```python
from build123d import *

# Parameters (mm, degrees)
BOSS_EXTRUDE3_DEPTH = 117
SKETCH3_W           = 2.281994321
SKETCH3_H           = 23.79794077
SKETCH3_W_2         = 80.521799592
SKETCH3_H_2         = 88.019780931
CUT_EXTRUDE1_DEPTH  = 117
SKETCH4_W           = 94.510648664
SKETCH4_H           = 87.992672894
CUT_EXTRUDE2_DEPTH  = 117


with BuildPart() as part:
    # Sketch2 → Boss-Extrude3 (new body)
    with BuildSketch(Plane(origin=(0, 0, 0), x_dir=(1, 0, 0), z_dir=(0, 1, 0))):
        Polygon((-826.128986822, -44.396477746), (-786.035151567, -12.233698412), (-620.035151567, -12.233698412), (-580.129096878, -44.629173391), (-580.129096878, -114.629173391), (-664.384727068, -191.421027004), (-742.086028689, -191.421027004), (-826.128986822, -114.396477746), align=None)
    extrude(amount=BOSS_EXTRUDE3_DEPTH)

    # Sketch3 → Cut-Extrude1 (cut)
    with BuildSketch(Plane(origin=(-206.167073408, 0, -226.205461612), x_dir=(0.7390844753537593, 0, -0.6736127509860976), z_dir=(0.6736127509860976, 0, 0.7390844753537593))):
        with Locations((-598.858942552, 121.091844218)):
            Rectangle(SKETCH3_W, SKETCH3_H)
        with Locations((-562.673032613, 60.618994727)):
            Rectangle(SKETCH3_W_2, SKETCH3_H_2)
    extrude(amount=-CUT_EXTRUDE1_DEPTH, mode=Mode.SUBTRACT)

    # Sketch4 → Cut-Extrude2 (cut)
    with BuildSketch(Plane(origin=(-434.116139586, 0, 473.672418674), x_dir=(0.7372189309889005, 0, 0.6756539408540315), z_dir=(-0.6756539408540315, 0, 0.7372189309889005))):
        with Locations((-474.328289605, 59.966544548)):
            Rectangle(SKETCH4_W, SKETCH4_H)
    extrude(amount=-CUT_EXTRUDE2_DEPTH, mode=Mode.SUBTRACT)


solid = part.part
```
Can you work these out from the model? Positions are in its coordinate system, mm. A direction names the side the tool comes from. Give positions to 0.01 mm unless a question says otherwise; leave off trailing zeros. Loops run counter-clockwise (first coordinate to the right, second up) from the corner with the lowest first, then second, coordinate; pieces in that order, holes last. Notation, with made-up numbers: M 84,23.5 L 133,23.5 A26 ccw 133,50.5 Z; hole C -3,54.5 d9. An arc over 180 degrees is marked long. Use one line per item in the form item = value. Start each with the question number.
(1) I want a section at D-D, the plane z = 140.5. Write out the boundary of the cut face in (x, y).
(2) Thinking about a two-plate mould opening in Z: for faces 1 (the flat face through (-754, 103.963, 120)), 2 (the flat face through (-703, 58, 191.421)), 3 (the flat face through (-688.03, 61.24, 54.67)), 4 (the flat face through (-826.129, 58, 80)), which applies, released by +Z, released by -Z, zero draft, split by the parting line, or undercut?
(3) I'm going to push flat-ended pins straight in: P1, Ø10, axis at x = -625, z = 56.5, coming from the -Y side; P2, Ø6, axis at y = 27, z = 39.5, coming from the +X side; P3, Ø12, axis at x = -637.5, y = 42, coming from the +Z side. Where does each tip first touch, or does it pass through?
(4) I want a section at A-A, the plane z = 76.5. Write out the boundary of the cut face in (x, y).
(5) I want a section at B-B, the plane x = -716. Write out the boundary of the cut face in (y, z).
(6) I want a section at C-C, the plane y = 40. Write out the boundary of the cut face in (x, z), and give its area (3 significant figures).
(7) On a 3-axis mill with a long thin cutter (end or side, diameter ignored), from which of +Z, -Z, +X, -X, +Y, -Y can I reach the whole of each face in a straight line? I mean faces 5 (the flat face through (-701, 0, 101)), 6 (the flat face through (-661, 104.629, 111)), 7 (the flat face through (-688, 109.193, 135)). Say none if no direction works.
(8) Please list where these lines run through material, in increasing order: line 1 (Y direction, x = -648, z = 112); line 2 (Y direction, x = -735, z = 136); line 3 (X direction, y = 97, z = 52.5).
Worked out:
q1.outline = M -797.65,0 L -608.51,0 L -608.51,16.61 L -687.73,16.61 L -687.73,104.63 L -608.51,104.63 L -608.51,117 L -680.67,117 L -680.67,109.19 L -683.76,109.19 L -683.76,117 L -797.65,117 L -797.65,103.96 L -708.07,103.96 L -708.07,15.97 L -797.65,15.97 Z
q2.face_1 = undercut
q2.face_2 = released by +Z
q2.face_3 = undercut
q2.face_4 = zero draft
q3.P1 = 0
q3.P2 = -582.75
q3.P3 = 82.66
q4.outline = M -826.13,0 L -580.13,0 L -580.13,117 L -826.13,117 Z; hole M -777.61,15.97 L -694.31,15.97 L -694.31,16.61 L -637.11,16.61 L -637.11,104.63 L -711.98,104.63 L -711.98,103.96 L -777.61,103.96 Z
q5.outline = M 0,12.23 L 117,12.23 L 117,101.74 L 109.19,101.74 L 109.19,105.13 L 117,105.13 L 117,191.42 L 0,191.42 Z; hole M 15.97,56.62 L 103.96,56.62 L 103.96,80.16 L 104.63,80.16 L 104.63,109.48 L 103.96,109.48 L 103.96,149.15 L 15.97,149.15 Z
q6.outline = M -826.13,44.4 L -786.04,12.23 L -620.04,12.23 L -580.13,44.63 L -580.13,114.63 L -592.27,125.7 L -671.09,39.23 L -703.12,68.42 L -739.59,35.01 L -818.64,121.26 L -826.13,114.4 Z; M -748.96,185.12 L -697.87,129.37 L -651.79,179.94 L -664.38,191.42 L -742.09,191.42 Z
q6.area = 17,700 mm²
q7.face_5 = +Z, -Z, +X, -X, -Y
q7.face_6 = none
q7.face_7 = +Y
q8.line_1 = 0 to 16.61, 104.63 to 117
q8.line_2 = 0 to 15.97, 103.96 to 117
q8.line_3 = -826.13 to -755.62, -720.5 to -685.65, -658.99 to -580.13
